Design review of the part built by this model. Coordinates are the model's own, in mm. A direction names the side the tool comes from. Coordinates: 2 decimals unless noted, no trailing zeros. Loops run counter-clockwise (first coordinate to the right, second up) from the corner with the lowest first, then second, coordinate; pieces in that order, holes last. Notation, with made-up numbers: (-35.5, -19) -> (-15.5, -19) arc R25 ccw to (-15.5, 3) -> close; hole circle Ø9 at (84.5, 72). An arc over 180 degrees is marked (long way). Use CSV: the item, a comma, the result in double quotes.
```python
from build123d import *

# Parameters (mm, degrees)
CHAMFER1_SIZE = 1
SKETCH2_W     = 1
SKETCH2_H     = 1


with BuildPart() as part:
    # Sketch1 → Revolve1 (revolve)
    with BuildSketch(Plane.XY):
        Polygon((0, 0), (0, 8), (-30, 8), (-30, 4), (-40, 4), (-40, 0), align=None)
    revolve(axis=Axis((-114.784060064, 0, 0), (1, 0, 0)))

    # Chamfer1
    chamfer1_edges = [part.edges().sort_by_distance(p)[0] for p in [
        (-40, -4, 0),
        (0, -8, 0),
    ]]
    chamfer(chamfer1_edges, length=CHAMFER1_SIZE)

    # Sketch2 → Cut-Revolve1 (revolve, cut)
    with BuildSketch(Plane.XY):
        with Locations((-30.5, 3.5)):
            Rectangle(SKETCH2_W, SKETCH2_H)
    revolve(axis=Axis((0, 0, 0), (-1, 0, 0)), mode=Mode.SUBTRACT)


solid = part.part
```
Item 1: To check wall thickness, follow line 1 along X through (y, z) = (-2, -5); line 2 along X through (y, z) = (-3.5, -1.75); line 3 along X through (y, z) = (3.5, -1.5). State the ranges of each line that lie inside material, in increasing order.
Checked values:
line 1,"-30 to 0"
line 2,"-39.09 to -31, -30 to 0"
line 3,"-39.19 to -31, -30 to 0"
Item 2: Machinability: for faces 1 (the face through (0, 0, 0)), 2 (the face through (-30, 3.4, 0.1)), 3 (the face through (-35.056, -0.867, -3.905)), which of the approach directions +Z, -Z, +X, -X, +Y, -Y give a long, thin tool a straight path to every point of the face, cutting with its end or side? Answer none if there is none.
Checked values:
face 1,"+Z, -Z, +X, +Y, -Y"
face 2,"none"
face 3,"-X"
Item 3: Draft analysis for pull direction X (two halves, no side actions). For faces 4 (the face through (-30.5, -3, -0.1)), 5 (the face through (-31, -1, -3)), 6 (the face through (-40, 0, 0)), 7 (the face through (-15.7, -1.73, -7.81)), state which applies: pulls with the +X half, pulls with the -X half, needs draft (parallel to the pull), parting line crosses it, or undercut.
Checked values:
face 4,"undercut"
face 5,"undercut"
face 6,"pulls with the -X half"
face 7,"needs draft"
Item 4: Add section C-C (x = -19.5). Give the boundary of the cut face in (y, z), then the cut area to 3 significant figures.
Checked values:
outline,"circle Ø16 at (0, 0)"
area,"201 mm^2"
Item 5: Add section A-A (y = 0). Give the boundary of the cut face in (x, z), then the cut area to 3 significant figures.
Checked values:
outline,"(-40, -3) -> (-39, -4) -> (-31, -4) -> (-31, -3) -> (-30, -3) -> (-30, -8) -> (-1, -8) -> (0, -7) -> (0, 7) -> (-1, 8) -> (-30, 8) -> (-30, 3) -> (-31, 3) -> (-31, 4) -> (-39, 4) -> (-40, 3) -> close"
area,"556 mm^2"
Item 6: Add section D-D (x = -36.5). Give the boundary of the cut face in (y, z).
Checked values:
outline,"circle Ø8 at (0, 0)"
Item 7: Clearance check with flat-ended pins moving along their axes: pin 1 (2 mm diameter, centred on x = -16, y = 2.5, fed in from -Z); pin 2 (4 mm diameter, centred on x = -27, y = -5.5, fed in from +Z). State where each tip first meets the part, or that it passes through.
Checked values:
pin 1,"z = -7.86"
pin 2,"z = 7.19"
